```python
from build123d import *

# Parameters (mm, degrees)
CYLINDER004_R     = 1.7
CYLINDER004_DEPTH = 6.5
CYLINDER002_R     = 3
CYLINDER002_DEPTH = 6.5
CYLINDER_R        = 26.5
CYLINDER_DEPTH    = 30
CYLINDER001_R     = 27.8
CYLINDER001_DEPTH = 30
CYLINDER005_R     = 1.7
CYLINDER005_DEPTH = 6.5
CYLINDER003_R     = 3
CYLINDER003_DEPTH = 6.5
CHAMFER_SIZE      = 1
FILLET_R          = 1


with BuildPart() as obj1:
    # Cylinder004 → Cylinder004 (new body)
    with BuildSketch(Plane(origin=(2.2, 8, -3.4), x_dir=(1, 0, 0), z_dir=(0, 0, 1))):
        Circle(CYLINDER004_R)
    extrude(amount=CYLINDER004_DEPTH)


with BuildPart() as cut001:
    # Cylinder002 → Cylinder002 (new body)
    with BuildSketch(Plane(origin=(2.2, 8, -2.8), x_dir=(1, 0, 0), z_dir=(0, 0, 1))):
        Circle(CYLINDER002_R)
    extrude(amount=CYLINDER002_DEPTH)

    # Cut001: cut obj1
    add(obj1.part, mode=Mode.SUBTRACT)


with BuildPart() as cut001_1:
    # Cut001 placement: moved
    add(cut001.part.moved(Location((0, 0, 16))))


with BuildPart() as base_exterior_vaciado:
    # Cylinder → Cylinder (new body)
    with BuildSketch(Plane(origin=(-12.5, 19, -10.6), x_dir=(1, 0, 0), z_dir=(0, 0, 1))):
        Circle(CYLINDER_R)
    extrude(amount=CYLINDER_DEPTH)


with BuildPart() as cut:
    # Cylinder001 → Cylinder001 (new body)
    with BuildSketch(Plane(origin=(-12.5, 19, -10), x_dir=(1, 0, 0), z_dir=(0, 0, 1))):
        Circle(CYLINDER001_R)
    extrude(amount=CYLINDER001_DEPTH)

    # Cut: cut base exterior vaciado
    add(base_exterior_vaciado.part, mode=Mode.SUBTRACT)


with BuildPart() as obj2:
    # Cylinder005 → Cylinder005 (new body)
    with BuildSketch(Plane(origin=(-29.1, 29.1, -3.4), x_dir=(1, 0, 0), z_dir=(0, 0, 1))):
        Circle(CYLINDER005_R)
    extrude(amount=CYLINDER005_DEPTH)


with BuildPart() as obj3:
    # Cylinder003 → Cylinder003 (new body)
    with BuildSketch(Plane(origin=(-29.1, 29.1, -2.8), x_dir=(1, 0, 0), z_dir=(0, 0, 1))):
        Circle(CYLINDER003_R)
    extrude(amount=CYLINDER003_DEPTH)

    # Cut002: cut obj2
    add(obj2.part, mode=Mode.SUBTRACT)


with BuildPart() as obj3_1:
    # Cut002 placement: moved
    add(obj3.part.moved(Location((0, 0, 16))))

    # Fusion: union Cut001, Cut
    add(cut001_1.part)
    add(cut.part)

    # Chamfer
    chamfer_edges = [obj3_1.edges().sort_by_distance(p)[0] for p in [
        (-32.1, 29.1, 19.4),
        (-39, 19, 19.4),
        (-0.8, 8, 19.4),
    ]]
    chamfer(chamfer_edges, length=CHAMFER_SIZE)

    # Fillet
    fillet_edges = [obj3_1.edges().sort_by_distance(p)[0] for p in [
        (-40.3, 19, 20),
    ]]
    fillet(fillet_edges, radius=FILLET_R)


solid = obj3_1.part
```
Model file for the job. Use its own axes, mm. A direction names the side the tool comes from. Coordinates: 2 decimals unless noted, no trailing zeros. Loops run counter-clockwise (first coordinate to the right, second up) from the corner with the lowest first, then second, coordinate; pieces in that order, holes last. Notation, with made-up numbers: (7, -7.5) - (19, -7.5) arc R30 ccw to (19, 27.5) - close; hole circle Ø2 at (-30.5, -19). An arc over 180 degrees is marked (long way). Write item = value, one per line. Start each with the question number.
Item 1: Saw through at D-D, the plane z = -1. List the corners of the cut face in (x, y).
Item 2: 3-axis set-ups, long thin cutter, end or side, ignore diameter. For faces 1 (the face through (-13, 19, 20)), 2 (the face through (-13, 19, 19.4)): which of +Z, -Z, +X, -X, +Y, -Y reach the whole face in a straight line?
Item 3: Saw through at B-B, the plane y = 19. List the corners of the cut face in (x, z).
Item 4: Drop flat-ended pins along their axis: pin 1 Ø3 at (x, y) = (3.5, 7.5) entering from -Z; pin 2 Ø4 at (x, z) = (-32, 4.5) entering from -Y; pin 3 Ø1 at (x, y) = (2.5, 7.5) entering from -Z. Give the stop position or say it passes through.
Item 5: Wall check: probe 1 along Y at (x, z) = (2, 17); probe 2 along Y at (x, z) = (-12.5, -2.75); probe 3 along X at (y, z) = (29, 17). Give the ranges that are in metal, low to high. Write a range as [from, to].
Item 6: Saw through at C-C, the plane x = -12.5. List the corners of the cut face in (y, z), then the cut area to 3 significant figures.
Item 7: Saw through at A-A, the plane z = 17. List the corners of the cut face in (x, y), then the cut area to 3 significant figures.
Item 8: Pull direction Y, two halves, no side cores. Call faces 3 (the face through (13.2, 8.4, 4.3)), 4 (the face through (12.776, 26.96, 4.001)), 5 (the face through (-2, -6, -10)): +Y half, -Y half, draft (parallel to the pull), parting line (faces both ways), or undercut.
Answers:
q1.outline = circle Ø55.6 at (-12.5, 19); hole circle Ø53 at (-12.5, 19)
q2.face_1 = +Z, +X, -X, +Y, -Y
q2.face_2 = -Z
q3.outline = (-40.3, -10) - (-39, -10) - (-39, 18.4) - (-38, 19.4) - (13, 19.4) - (14, 18.4) - (14, -10) - (15.3, -10) - (15.3, 19) arc R1 ccw to (14.3, 20) - (-39.3, 20) arc R1 ccw to (-40.3, 19) - close
q4.pin_1 = 13.2
q4.pin_2 = -2.6
q4.pin_3 = 19.1
q5.probe_1 = [-4.72, -3.18], [5.01, 6.31], [9.69, 10.99], [41.18, 42.72]
q5.probe_2 = [-8.8, -7.5], [45.5, 46.8]
q5.probe_3 = [-38.44, -37.04], [-32.1, -30.8], [-27.4, -26.1], [12.04, 13.44]
q6.outline = (-8.8, -10) - (-7.5, -10) - (-7.5, 18.4) - (-6.5, 19.4) - (44.5, 19.4) - (45.5, 18.4) - (45.5, -10) - (46.8, -10) - (46.8, 19) arc R1 ccw to (45.8, 20) - (-7.8, 20) arc R1 ccw to (-8.8, 19) - close
q6.area = 110 mm2
q7.outline = circle Ø55.6 at (-12.5, 19); circle Ø6 at (-29.1, 29.1); circle Ø6 at (2.2, 8); hole circle Ø53 at (-12.5, 19); hole circle Ø3.4 at (-29.1, 29.1); hole circle Ø3.4 at (2.2, 8)
q7.area = 260 mm2
q8.face_3 = parting line
q8.face_4 = undercut
q8.face_5 = draft
